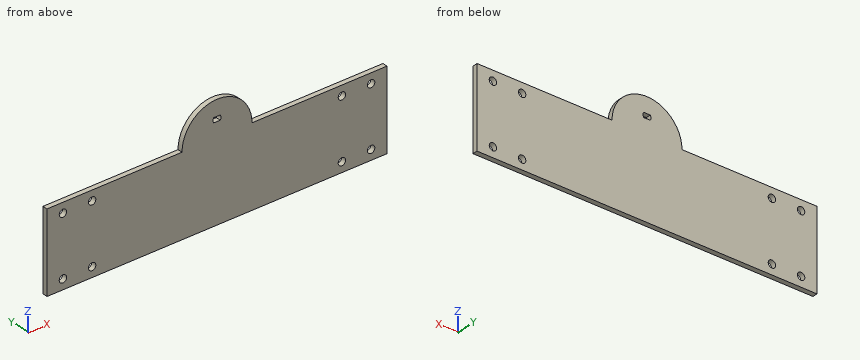
```python
from build123d import *

# Parameters (mm, degrees)
BOSS_EXTRUDE1_DEPTH = 3.175
SKETCH2_R           = 2.3495
CUT_EXTRUDE1_DEPTH  = 4.175


with BuildPart() as part:
    # Sketch1 → Boss-Extrude1 (new body)
    with BuildSketch(Plane(origin=(0, 0, 0), x_dir=(1, 0, 0), z_dir=(0, 1, 0))):
        with BuildLine():
            Line((-107.95, 61.595), (107.95, 61.595))
            Line((107.95, 61.595), (107.95, 10.795))
            Line((107.95, 10.795), (22.225, 10.795))
            ThreePointArc((22.225, 10.795), (0, -11.43), (-22.225, 10.795))
            Line((-22.225, 10.795), (-107.95, 10.795))
            Line((-107.95, 10.795), (-107.95, 61.595))
        make_face()
        with BuildLine():
            Line((-2.032, 1.524), (2.032, 1.524))
            ThreePointArc((2.032, 1.524), (2.54, 0), (2.032, -1.524))
            Line((2.032, -1.524), (-2.032, -1.524))
            ThreePointArc((-2.032, -1.524), (-2.54, 0), (-2.032, 1.524))
        make_face(mode=Mode.SUBTRACT)
    extrude(amount=BOSS_EXTRUDE1_DEPTH)

    # Sketch2 → Cut-Extrude1 (cut, through all)
    with BuildSketch(Plane(origin=(0, 3.175, 0), x_dir=(1, 0, 0), z_dir=(0, 1, 0))):
        with Locations((-97.8535, 55.245)):
            Circle(SKETCH2_R)
        with Locations((-97.8535, 17.145)):
            Circle(SKETCH2_R)
        with Locations((-79.3115, 17.145)):
            Circle(SKETCH2_R)
        with Locations((-79.3115, 55.245)):
            Circle(SKETCH2_R)
        with Locations((79.3115, 55.245)):
            Circle(SKETCH2_R)
        with Locations((79.3115, 17.145)):
            Circle(SKETCH2_R)
        with Locations((97.8535, 17.145)):
            Circle(SKETCH2_R)
        with Locations((97.8535, 55.245)):
            Circle(SKETCH2_R)
    extrude(amount=-CUT_EXTRUDE1_DEPTH, mode=Mode.SUBTRACT)


solid = part.part
```
Design review of the part built by this model. Coordinates are the model's own, in mm. Give positions to 0.01 mm unless a question says otherwise; leave off trailing zeros. Order: outer loops, then holes, each group sorted by start corner. A loop starts at its lowest first (then second) coordinate and runs counter-clockwise, first axis right, second up. Notation, with made-up numbers: (6.25, 1) - (55.25, 1) arc R26 ccw to (55.25, 15) - close; hole circle Ø11 at (0.25, 62.25). An arc over 180 degrees is marked (long way). Use a Markdown table: item, result. Add a question column.
(1) Add section C-C on x = 86. Give the boundary of the cut face in (y, z) (3 decimals), then the cut area to 3 significant figures.
(2) Add section A-A on x = 0. Give the boundary of the cut face in (y, z) (3 decimals).
(3) Wall thickness on probe 1 along Z at (x, y) = (63, 3.05) (3 decimals); probe 2 along X at (y, z) = (0.4, -7); probe 3 along Z at (x, y) = (-19, 1.55) (3 decimals): over which ranges is each line inside the solid? List them lowest first. Write a range as [from, to].
(4) Clearance check with flat-ended pins moving along their axes: P1, Ø1.5, axis at x = 19.5, z = -4.5, coming from the -Y side; P2, Ø1, axis at x = 77, y = 1.5, coming from the +Z side (3 decimals); P3, Ø1, axis at x = 0, y = 2.5, coming from the +Z side. State where each tip first meets the part, or that it passes through.
(5) Add section B-B on y = 1.9. Give the number of separate pieces and of enclosed holes in the cut face, then the cut area to 3 significant figures.
Report:
| question | item | result |
|---|---|---|
| 1 | outline | (0, -61.595) - (3.175, -61.595) - (3.175, -10.795) - (0, -10.795) - close |
| 1 | area | 161 mm² |
| 2 | outline | (0, -61.595) - (3.175, -61.595) - (3.175, -1.524) - (0, -1.524) - close; (0, 1.524) - (3.175, 1.524) - (3.175, 11.43) - (0, 11.43) - close |
| 3 | probe 1 | z = [-61.595, -10.795] |
| 3 | probe 2 | x = [-21.9, 21.9] |
| 3 | probe 3 | z = [-61.595, 0.735] |
| 4 | P1 | stops at y = 0 |
| 4 | P2 | stops at z = -10.795 |
| 4 | P3 | stops at z = 11.43 |
| 5 | separate pieces | 1 |
| 5 | enclosed holes | 9 |
| 5 | area | 11,600 mm² |
